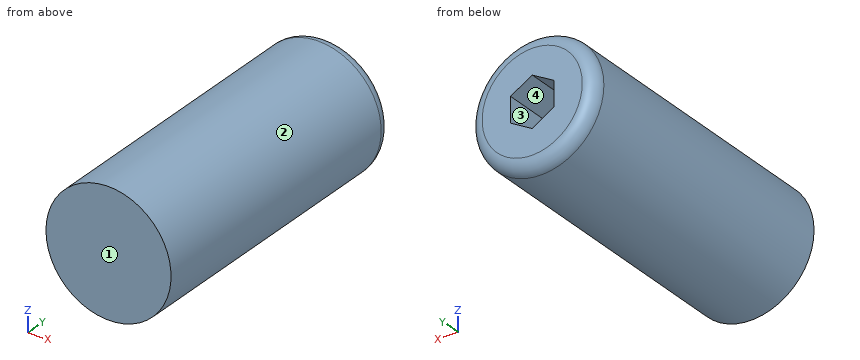
Autodesk Inventor part; units mm, degrees
ref_plane "YZ Plane" through (0, 0, 0) normal (1, 0, 0) x (0, 1, 0)
ref_plane "XZ Plane" through (0, 0, 0) normal (0, 1, 0) x (-1, 0, 0)
ref_plane "XY Plane" through (0, 0, 0) normal (0, 0, 1) x (1, 0, 0)
sketch "Sketch1" plane through (0, 0, 0) normal (0, 1, 0) x (-1, 0, 0)
  circle A0 centre (0, 0) radius 2.5
  dimension "d0" = 5
extrude "Extrusion1" add sketch "Sketch1" along normal blind 12
fillet "Fillet1" radius 0.5 1 edges at (2.5, 12, 0)
sketch "Sketch2" plane through (0, 12, 0) normal (0, 1, 0) x (1, 0, 0)
  line L0 (0, 1) -> (0.866, 0.5)
  line L1 (0.866, 0.5) -> (0.866, -0.5)
  line L2 (0.866, -0.5) -> (0, -1)
  line L3 (0, -1) -> (-0.866, -0.5)
  line L4 (-0.866, -0.5) -> (-0.866, 0.5)
  line L5 (-0.866, 0.5) -> (0, 1)
  point P0 (0, 0)
  point P1 (0, 0)
  dimension "d4" = 1
extrude "Extrusion2" cut sketch "Sketch2" against normal blind 2
properties part number "5mm Screw"
Geometry check sheet. Reference: the model listing, model coordinates, mm. Face numbers are marked on the shaded views. Coordinates: 2 decimals unless noted, no trailing zeros. Order: outer loops, then holes, each group sorted by start corner. A loop starts at its lowest first (then second) coordinate and runs counter-clockwise, first axis right, second up. Notation, with made-up numbers: (11.25, 28.25) - (60.25, 28.25) arc R16 cw to (60.25, 52.25) - close; hole circle Ø4 at (87, 67). An arc over 180 degrees is marked (long way). Answer in a Markdown table with one row per item. Add a question column.
1. Section check B-B (y = 6). Enter the section's corners in (x, z).
2. Material ranges on L1, parallel to Y at x = 0.45, z = -0.65; L2, parallel to X at y = 10.5, z = 0.4; L3, parallel to Z at x = 0.3, y = 0.5, recorded low to high. Write a range as [from, to].
3. Gauge pin test, flat ends, axial feed: pin 1 Ø1.5 at (x, y) = (-1.5, 10.5) entering from +Z; pin 2 Ø1.5 at (y, z) = (1.5, 2) entering from -X. Record the tip position at first contact, or that the pin passes through.
4. Draft check along X on the marked faces 1, 2, 3 and 4. Enter one of: +X half, -X half, draft (parallel to the pull), parting line (faces both ways), or undercut.
5. Section check A-A (z = 0). Enter the section's corners in (x, y).
Data:
| question | item | result |
|---|---|---|
| 1 | outline | circle Ø5 at (0, 0) |
| 2 | L1 | y = [0, 10] |
| 2 | L2 | x = [-2.47, -0.87], [0.87, 2.47] |
| 2 | L3 | z = [-2.48, 2.48] |
| 3 | pin 1 | stops at z = 2.38 |
| 3 | pin 2 | stops at x = -2.17 |
| 4 | face 1 | draft |
| 4 | face 2 | parting line |
| 4 | face 3 | undercut |
| 4 | face 4 | undercut |
| 5 | outline | (-2.5, 0) - (2.5, 0) - (2.5, 11.5) arc R0.5 ccw to (2, 12) - (0.87, 12) - (0.87, 10) - (-0.87, 10) - (-0.87, 12) - (-2, 12) arc R0.5 ccw to (-2.5, 11.5) - close |
